Geometry check sheet. Reference: the model listing, model coordinates, mm. Face numbers are marked on the shaded views. A direction names the side the tool comes from. Coordinates: 2 decimals unless noted, no trailing zeros. Write each loop counter-clockwise with the first axis right and the second up, starting at its lowest first coordinate (ties: lowest second). Pieces come first, ordered by that corner, then holes. Notation, with made-up numbers: M 76,26 L 132,26 A36 ccw 132,63 Z; hole C 43.5,24.5 d2. An arc over 180 degrees is marked long. Write item = value, one per line. Start each with the question number.
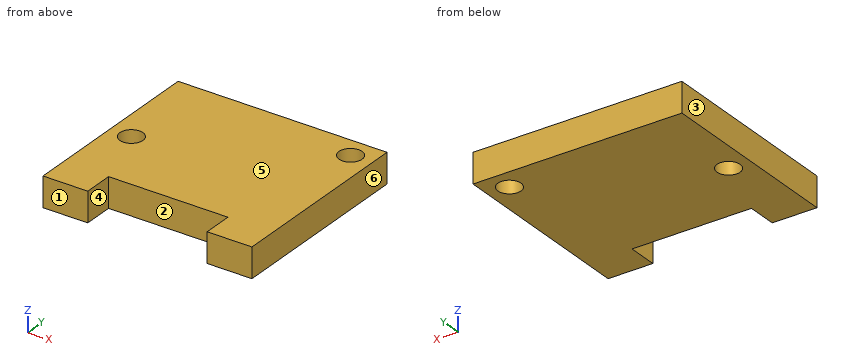
Autodesk Inventor part; units mm, degrees
ref_plane "YZ Plane" through (0, 0, 0) normal (1, 0, 0) x (0, 1, 0)
ref_plane "XZ Plane" through (0, 0, 0) normal (0, 1, 0) x (-1, 0, 0)
ref_plane "XY Plane" through (0, 0, 0) normal (0, 0, 1) x (1, 0, 0)
sketch "Sketch1" plane through (0, 0, 0) normal (0, 0, 1) x (1, 0, 0)
  line L0 (-14, 0) -> (14, 0)
  line L1 (14, 0) -> (14, 16)
  line L2 (14, 16) -> (-14, 16)
  line L3 (-14, 16) -> (-14, 0)
  circle A0 centre (-11.1, 2.85) radius 1.55
  circle A1 centre (11.1, 13.15) radius 1.55
  line L4 (-11.1, 2.85) -> (-14, 2.85) construction
  line L5 (11.1, 13.15) -> (14, 13.15) construction
  line L6 (11.1, 13.15) -> (11.1, 16) construction
  line L7 (-11.1, 2.85) -> (-11.1, 0) construction
  line L8 (-14, 0) -> (14, 0) construction
  line L9 (14, 0) -> (14, -6)
  line L10 (14, -6) -> (8, -6) construction
  line L11 (-14, -6) -> (-14, 0)
  line L12 (-14, -6) -> (-8, -6) construction
  line L13 (-8, -6) -> (-8, -10)
  line L14 (-8, -10) -> (-14, -10)
  line L15 (-14, -10) -> (-14, -6)
  line L16 (14, -6) -> (8, -6) construction
  line L17 (8, -6) -> (8, -10)
  line L18 (8, -10) -> (14, -10)
  line L19 (14, -10) -> (14, -6)
  line L20 (-8, -6) -> (-14, -6) construction
  line L21 (8, -6) -> (-8, -6)
  point P0 (0, 0)
  point P1 (0, 0)
  point P2 (14, 0)
  point P3 (14, 0)
  dimension "d0" = 3.1
  dimension "d1" = 22.2
  dimension "d2" = 10.3
  dimension "d3" = 16
  dimension "d4" = 28
  dimension "d5" = 22
  dimension "d8" = 6
  dimension "d9" = 6
  dimension "d10" = 4
extrude "Extrusion1" add sketch "Sketch1" along normal blind 4
properties part number "SwitchHolder_V2" material "Wood (Oak)"
Q1. Set-up check for the marked faces 1 and 2: record each of +Z, -Z, +X, -X, +Y, -Y from which the full face is reachable in a straight line by a thin tool's end or side.
Q2. Draft check along X on the marked faces 3, 4, 5 and 6. Enter one of: pulls with the +X half, pulls with the -X half, needs draft (parallel to the pull), parting line crosses it, or undercut.
Q3. Gauge pin test, flat ends, axial feed: pin 1 (2 mm diameter, centred on x = 4, z = 2.5, fed in from -Y); pin 2 (2.5 mm diameter, centred on x = 11.1, y = 13.15, fed in from -Z). Record the tip position at first contact, or that the pin passes through.
Q4. Scan lines: L1, parallel to Y at x = 11.1, z = 2; L2, parallel to Y at x = -11.1, z = 1.9; L3, parallel to Y at x = 5.25, z = 0.4. Record each from-to range of solid material in increasing order.
Q5. Cross-section at C-C on z = 1.5. Enter the section's corners in (x, y).
Q6. Cross-section at D-D on x = -3.25. Enter the section's corners in (y, z), and give its area (3 significant figures).
Q7. Cross-section at B-B on x = -11.1. Enter the section's corners in (y, z).
Q8. Cross-section at A-A on y = 13.15. Enter the section's corners in (x, z), and give its area (3 significant figures).
Values found:
q1.face_1 = +Z, -Z, +X, -X, -Y
q1.face_2 = +Z, -Z, -Y
q2.face_3 = pulls with the -X half
q2.face_4 = undercut
q2.face_5 = needs draft
q2.face_6 = pulls with the +X half
q3.pin_1 = -6
q3.pin_2 = through
q4.L1 = -10 to 11.6, 14.7 to 16
q4.L2 = -10 to 1.3, 4.4 to 16
q4.L3 = -6 to 16
q5.outline = M -14,-10 L -8,-10 L -8,-6 L 8,-6 L 8,-10 L 14,-10 L 14,16 L -14,16 Z; hole C -11.1,2.85 d3.1; hole C 11.1,13.15 d3.1
q6.outline = M -6,0 L 16,0 L 16,4 L -6,4 Z
q6.area = 88.0 mm²
q7.outline = M -10,0 L 1.3,0 L 1.3,4 L -10,4 Z; M 4.4,0 L 16,0 L 16,4 L 4.4,4 Z
q8.outline = M -14,0 L 9.55,0 L 9.55,4 L -14,4 Z; M 12.65,0 L 14,0 L 14,4 L 12.65,4 Z
q8.area = 99.6 mm²
